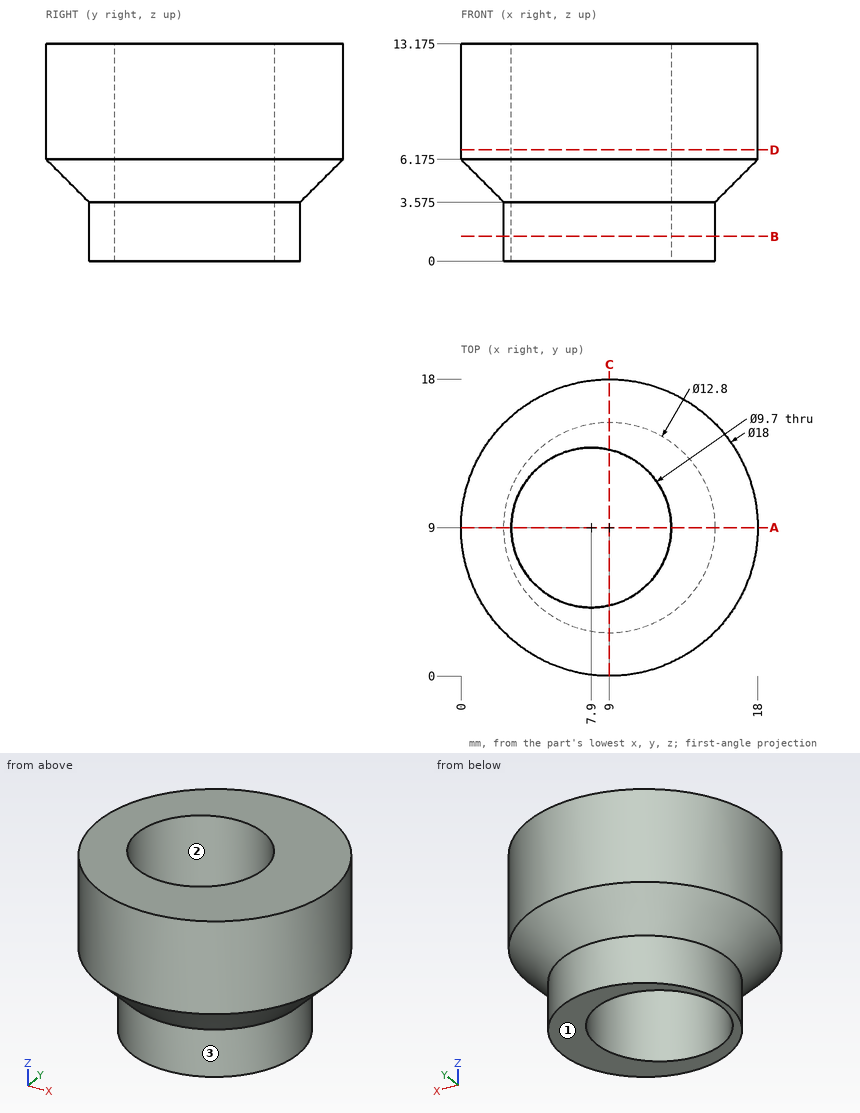
Verification items for this drawing (mm, ordinates from the low corner). Give positions to 0.01 mm unless a question says otherwise; leave off trailing zeros. Loops run counter-clockwise (first coordinate to the right, second up) from the corner with the lowest first, then second, coordinate; pieces in that order, holes last. Notation, with made-up numbers: M -9.5,32.25 L -1.5,32.25 A31 cw -1.5,63.25 Z; hole C -4,81.5 d6. An arc over 180 degrees is marked long. Return JSON: item names as keys, results as strings. Group by question number.
1. Cross-section at D-D on z = 6.75. Record the boundary of the cut face in (x, y), plus the area to 3 significant figures.
2. Thickness scan on L1, parallel to X at y = 9, z = 8.25; L2, parallel to Y at x = 4.5, z = 12.5; L3, parallel to Y at x = 12.25, z = 5.75. Record the ranges inside material, lowest first.
3. Cross-section at A-A on y = 9. Record the boundary of the cut face in (x, z) (3 decimals).
4. Cross-section at C-C on x = 9. Record the boundary of the cut face in (y, z) (3 decimals).
5. Cross-section at B-B on z = 1.5. Record the boundary of the cut face in (x, y), plus the area to 3 significant figures.
6. Mould release check, pull along X, two halves, no side actions. Record for the marked faces 1, 2 and 3: released by +X, released by -X, zero draft, split by the parting line, or undercut.
7. Go/stop test with flat-tipped pins: pin 1 (4 mm diameter, centred on y = 8, z = 3, fed in from +X); pin 2 (2 mm diameter, centred on x = 2.5, z = 2.5, fed in from +Y); pin 3 (1 mm diameter, centred on y = 13.5, z = 11, fed in from -X); pin 4 (1.5 mm diameter, centred on x = 10.5, y = 2.5, fed in from -Z). Record where each tip stops, or that it passes through.
Return value:
{
 "1": {"outline": "C 9,9 d18; hole C 7.9,9 d9.7", "area": "181 mm^2"},
 "2": {"L1": "0 to 3.05, 12.75 to 18", "L2": "1.21 to 5.54, 12.46 to 16.79", "L3": "1.06 to 6.86, 11.14 to 16.94"},
 "3": {"outline": "M 0,6.175 L 2.6,3.575 L 2.6,0 L 3.05,0 L 3.05,13.175 L 0,13.175 Z; M 12.75,0 L 15.4,0 L 15.4,3.575 L 18,6.175 L 18,13.175 L 12.75,13.175 Z"},
 "4": {"outline": "M 0,6.175 L 2.6,3.575 L 2.6,0 L 4.276,0 L 4.276,13.175 L 0,13.175 Z; M 13.724,0 L 15.4,0 L 15.4,3.575 L 18,6.175 L 18,13.175 L 13.724,13.175 Z"},
 "5": {"outline": "C 9,9 d12.8; hole C 7.9,9 d9.7", "area": "54.8 mm^2"},
 "6": {"face 1": "zero draft", "face 2": "undercut", "face 3": "split by the parting line"},
 "7": {"pin 1": "x = 16.77", "pin 2": "y = 12.27", "pin 3": "x = 0.94", "pin 4": "z = 0"}
}
